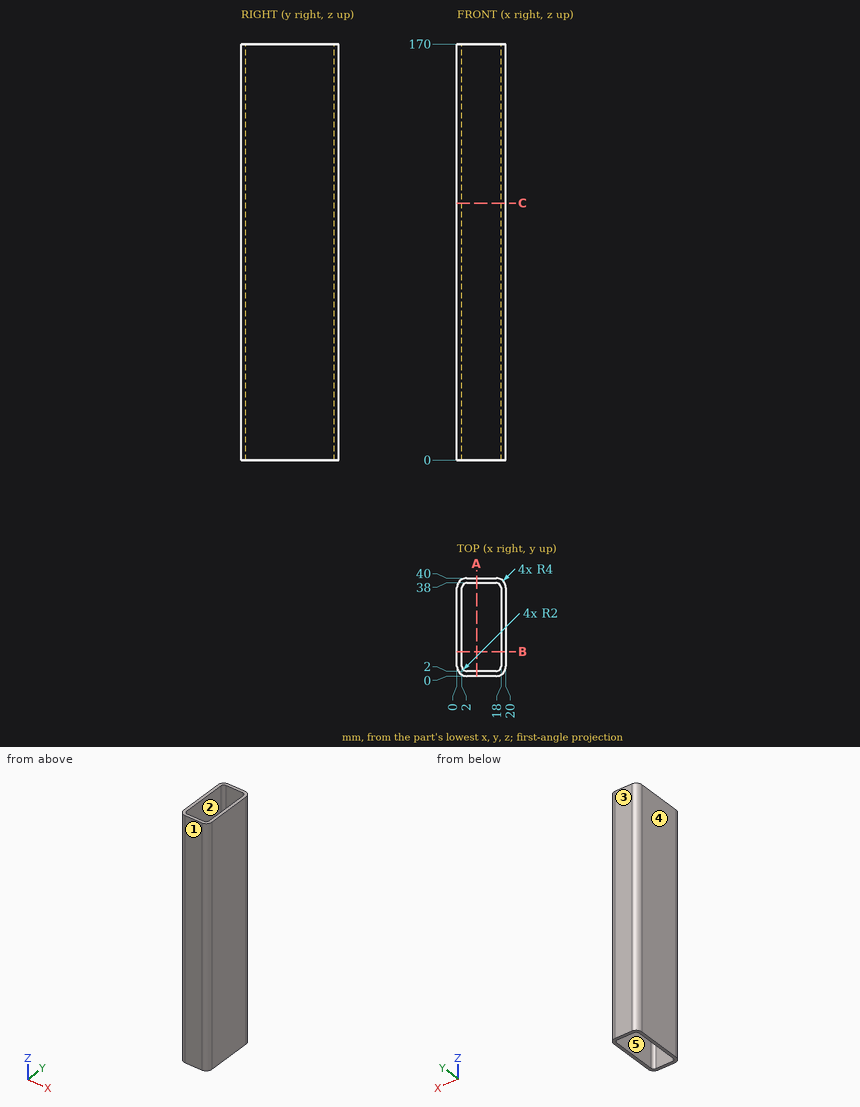
Verification items for this drawing (mm, ordinates from the low corner). A direction names the side the tool comes from. Give positions to 0.01 mm unless a question says otherwise; leave off trailing zeros. Write each loop counter-clockwise with the first axis right and the second up, starting at its lowest first coordinate (ties: lowest second). Pieces come first, ordered by that corner, then holes. Notation, with made-up numbers: (-37, 58.5) -> (21, 58.5) arc R32 ccw to (21, 86.5) -> close; hole circle Ø8 at (-8.75, -31.5). An arc over 180 degrees is marked (long way). Write item = value, one per line.
Item 1: Tool access check on the marked faces 1 and 2. Record the directions out of +Z, -Z, +X, -X, +Y, -Y that give a thin tool (end or side, any length) a straight path to the whole face; none if there is none.
Output:
face_1 = +Z, -Z, +X, -X, -Y
face_2 = +Z, -Z
Item 2: Sectioned sample at B-B on y = 10. Record the boundary of the cut face in (x, z).
Output:
outline = (0, 0) -> (2, 0) -> (2, 170) -> (0, 170) -> close; (18, 0) -> (20, 0) -> (20, 170) -> (18, 170) -> close
Item 3: Sectioned sample at C-C on z = 105. Record the boundary of the cut face in (x, y).
Output:
outline = (0, 4) arc R4 ccw to (4, 0) -> (16, 0) arc R4 ccw to (20, 4) -> (20, 36) arc R4 ccw to (16, 40) -> (4, 40) arc R4 ccw to (0, 36) -> close; hole (2, 4) arc R2 ccw to (4, 2) -> (16, 2) arc R2 ccw to (18, 4) -> (18, 36) arc R2 ccw to (16, 38) -> (4, 38) arc R2 ccw to (2, 36) -> close
Item 4: Release check for a two-part mould opening along X. For the marked faces 3, 4 and 5 record: +X half, -X half, draft (parallel to the pull), parting line (faces both ways), or undercut.
Output:
face_3 = draft
face_4 = -X half
face_5 = undercut
Item 5: Sectioned sample at A-A on x = 8. Record the boundary of the cut face in (y, z), and give its area (3 significant figures).
Output:
outline = (0, 0) -> (2, 0) -> (2, 170) -> (0, 170) -> close; (38, 0) -> (40, 0) -> (40, 170) -> (38, 170) -> close
area = 680 mm^2
Item 6: Scan lines: probe 1 along X at (y, z) = (34, 118); probe 2 along Y at (x, z) = (16.25, 120); probe 3 along Y at (x, z) = (16.5, 55). Record each from-to range of solid material in increasing order. Write a range as from..to.
Output:
probe_1 = 0..2, 18..20
probe_2 = 0.01..2.02, 37.98..39.99
probe_3 = 0.03..2.06, 37.94..39.97
Item 7: Gauge pin test, flat end, axial feed: pin 1 (1.5 mm diameter, centred on x = 3, z = 117.5, fed in from +Y). Record the tip position at first contact, or that the pin passes through.
Output:
pin_1 = 39.99
